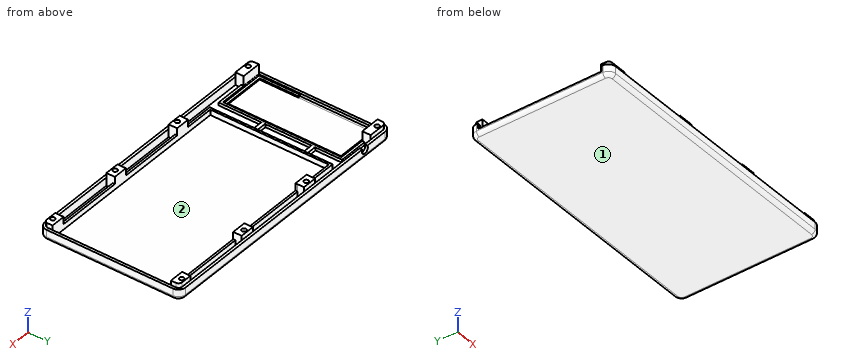
from build123d import *

# Parameters (mm, degrees)
ESQUISSE1_W             = 152.2
ESQUISSE1_H             = 78.4
BOSS_EXTRU_1_DEPTH      = 5.9
BOSS_EXTRU_2_DEPTH      = 1.4
BOSS_EXTRU_5_START      = 1.4
ESQUISSE1_5_R           = 1.25
BOSS_EXTRU_5_DEPTH      = 7
ESQUISSE1_5_W           = 8
ESQUISSE1_5_H           = 3.5
BOSS_EXTRU_5_2_DEPTH    = 7
BOSS_EXTRU_5_3_DEPTH    = 7
BOSS_EXTRU_5_4_DEPTH    = 7
BOSS_EXTRU_5_5_DEPTH    = 7
BOSS_EXTRU_5_6_DEPTH    = 7
BOSS_EXTRU_7_START      = 1.4
BOSS_EXTRU_7_DEPTH      = 3
CONG_1_R                = 4
CONG_4_R                = 2
BOSS_EXTRU_8_START      = 1.4
BOSS_EXTRU_8_DEPTH      = 0.75
BOSS_EXTRU_9_START      = 1.4
BOSS_EXTRU_9_DEPTH      = 1.65
BOSS_EXTRU_11_START     = 7
ESQUISSE4_R             = 1.25
BOSS_EXTRU_11_DEPTH     = 7
ESQUISSE5_W             = 6.6
ESQUISSE5_H             = 2
BOSS_EXTRU_12_DEPTH     = 2
CONG_3_R                = 2
ESQUISSE2_W             = 1.5
ESQUISSE2_H             = 68.8
ENL_V_MAT_EXTRU_1_DEPTH = 3
ENL_V_MAT_EXTRU_2_DEPTH = 1.5
ESQUISSE7_W             = 1.4
ESQUISSE7_H             = 41.680372202
ENL_V_MAT_EXTRU_3_DEPTH = 0.8
ESQUISSE8_W             = 7.99674486
ESQUISSE8_H             = 1.2
ESQUISSE8_W_2           = 8.000773141
ESQUISSE8_W_3           = 8
BOSS_EXTRU_13_DEPTH     = 4


with BuildPart() as part:
    # Esquisse1 → Boss.-Extru.1 (new body)
    with BuildSketch(Plane.XY):
        with Locations((74.6, 37.7)):
            Rectangle(ESQUISSE1_W, ESQUISSE1_H)
        with BuildLine():
            Line((0, 0), (147.2, 0))
            ThreePointArc((147.2, 0), (148.614213562, 0.585786438), (149.2, 2))
            Line((149.2, 2), (149.2, 73.4))
            ThreePointArc((149.2, 73.4), (148.614213562, 74.814213562), (147.2, 75.4))
            Line((147.2, 75.4), (0, 75.4))
            Line((0, 75.4), (0, 0))
        make_face(mode=Mode.SUBTRACT)
    extrude(amount=BOSS_EXTRU_1_DEPTH)

    # Esquisse1<4> → Boss.-Extru.2 (add)
    with BuildSketch(Plane.XY):
        with BuildLine():
            Line((0, 0), (147.2, 0))
            ThreePointArc((147.2, 0), (148.614213562, 0.585786438), (149.2, 2))
            Line((149.2, 2), (149.2, 73.4))
            ThreePointArc((149.2, 73.4), (148.614213562, 74.814213562), (147.2, 75.4))
            Line((147.2, 75.4), (0, 75.4))
            Line((0, 75.4), (0, 0))
        make_face()
    extrude(amount=BOSS_EXTRU_2_DEPTH)

    # Esquisse1<6> → Boss.-Extru.7 (add)
    with BuildSketch(Plane.XY.offset(BOSS_EXTRU_7_START)):
        Polygon((149.2, 70.7), (149.2, 71.9), (141.2, 71.9), (104.2, 71.9), (96.2, 71.9), (59.2, 71.9), (51.2, 71.9), (34, 71.9), (34, 37.7), (35.2, 37.7), (35.2, 70.7), align=None)
        Polygon((149.2, 3.5), (149.2, 4.7), (35.2, 4.7), (35.2, 37.7), (34, 37.7), (34, 3.5), (51.2, 3.5), (59.2, 3.5), (96.2, 3.5), (104.2, 3.5), (141.2, 3.5), align=None)
    extrude(amount=BOSS_EXTRU_7_DEPTH)

    # Congé1
    cong_1_edges = [part.edges().sort_by_distance(p)[0] for p in [
        (-1.5, 76.9, 2.95),
        (150.7, 76.9, 2.95),
        (150.7, -1.5, 2.95),
        (-1.5, -1.5, 2.95),
    ]]
    fillet(cong_1_edges, radius=CONG_1_R)

    # Congé4
    cong_4_edges = [part.edges().sort_by_distance(p)[0] for p in [
        (0, 75.4, 3.65),
        (0, 0, 3.65),
    ]]
    fillet(cong_4_edges, radius=CONG_4_R)

    # Esquisse1<7> → Boss.-Extru.8 (add)
    with BuildSketch(Plane.XY.offset(BOSS_EXTRU_8_START)):
        Polygon((24.6, 37.7), (26, 37.7), (26, 70.7), (0, 70.7), (0, 37.7), (1.4, 37.7), (1.4, 69.3), (24.6, 69.3), align=None)
        Polygon((26, 4.7), (26, 37.7), (24.6, 37.7), (24.6, 6.1), (1.4, 6.1), (1.4, 37.7), (0, 37.7), (0, 4.7), align=None)
    extrude(amount=BOSS_EXTRU_8_DEPTH)

    # Esquisse1<8> → Boss.-Extru.9 (add)
    with BuildSketch(Plane.XY.offset(BOSS_EXTRU_9_START)):
        Polygon((27.4, 3.3), (27.4, 72.1), (0, 72.1), (0, 70.7), (26, 70.7), (26, 4.7), (0, 4.7), (0, 3.3), align=None)
    extrude(amount=BOSS_EXTRU_9_DEPTH)

    # Esquisse4 → Boss.-Extru.11 (add)
    # profile 1 of 2: a face of its own
    with BuildSketch(Plane.XY.offset(1.4).offset(BOSS_EXTRU_11_START)):
        with BuildLine():
            Line((11, 75.4), (2, 75.4))
            ThreePointArc((2, 75.4), (0.585786438, 74.814213562), (0, 73.4))
            Line((0, 73.4), (0, 70.737356087))
            Line((0, 70.737356087), (11, 70.737356087))
            Line((11, 70.737356087), (11, 75.4))
        make_face()
        with Locations((4, 73.6)):
            Circle(ESQUISSE4_R, mode=Mode.SUBTRACT)
    # profile 2 of 2: a face of its own
    with BuildSketch(Plane.XY.offset(1.4).offset(BOSS_EXTRU_11_START)):
        with BuildLine():
            Line((0, 4.608067271), (11, 4.608067271))
            Line((11, 4.608067271), (11, 0))
            Line((11, 0), (2, 0))
            ThreePointArc((2, 0), (0.585786438, 0.585786438), (0, 2))
            Line((0, 2), (0, 4.608067271))
        make_face()
        with Locations((4, 1.8)):
            Circle(ESQUISSE4_R, mode=Mode.SUBTRACT)
    extrude(amount=-BOSS_EXTRU_11_DEPTH)

    # Esquisse5 → Boss.-Extru.12 (add)
    with BuildSketch(Plane.XY.offset(1.4)):
        with Locations((30.7, 56.329620473)):
            Rectangle(ESQUISSE5_W, ESQUISSE5_H)
        with Locations((30.7, 28.421993419)):
            Rectangle(ESQUISSE5_W, ESQUISSE5_H)
    extrude(amount=BOSS_EXTRU_12_DEPTH)

    # Congé3
    cong_3_edges = [part.edges().sort_by_distance(p)[0] for p in [
        (-1.5, 37.7, 0),
        (74.6, 76.9, 0),
        (150.7, 37.7, 0),
        (74.6, -1.5, 0),
        (149.528427125, 75.728427125, 0),
        (149.528427125, -0.328427125, 0),
        (-0.328427125, -0.328427125, 0),
        (-0.328427125, 75.728427125, 0),
    ]]
    fillet(cong_3_edges, radius=CONG_3_R)

    # Esquisse2 → Enlèv. mat.-Extru.1 (cut)
    with BuildSketch(Plane.XY.offset(5.9)):
        with Locations((-0.75, 37.7)):
            Rectangle(ESQUISSE2_W, ESQUISSE2_H)
    extrude(amount=-ENL_V_MAT_EXTRU_1_DEPTH, mode=Mode.SUBTRACT)

    # Esquisse6 → Enlèv. mat.-Extru.2 (cut)
    with BuildSketch(Plane(origin=(0, 76.9, 0), x_dir=(1, 0, 0), z_dir=(0, 1, 0))):
        with BuildLine():
            Line((17, -2.595457244), (17.25, -2.595457244))
            ThreePointArc((17.25, -2.595457244), (18.664213562, -3.181243681), (19.25, -4.595457244))
            Line((19.25, -4.595457244), (19.25, -4.845457244))
            ThreePointArc((19.25, -4.845457244), (18.664213562, -6.259670806), (17.25, -6.845457244))
            Line((17.25, -6.845457244), (17, -6.845457244))
            ThreePointArc((17, -6.845457244), (15.585786438, -6.259670806), (15, -4.845457244))
            Line((15, -4.845457244), (15, -4.595457244))
            ThreePointArc((15, -4.595457244), (15.585786438, -3.181243681), (17, -2.595457244))
        make_face()
    extrude(amount=-ENL_V_MAT_EXTRU_2_DEPTH, mode=Mode.SUBTRACT)

    # Esquisse7 → Enlèv. mat.-Extru.3 (cut)
    with BuildSketch(Plane.XY.offset(2.15)):
        with Locations((0.7, 48.459813899)):
            Rectangle(ESQUISSE7_W, ESQUISSE7_H)
    extrude(amount=-ENL_V_MAT_EXTRU_3_DEPTH, mode=Mode.SUBTRACT)



with BuildPart() as body_2:
    # Esquisse1<5> → Boss.-Extru.5 (new body)
    with BuildSketch(Plane.XY.offset(BOSS_EXTRU_5_START)):
        with BuildLine():
            Line((141.2, 71.9), (149.2, 71.9))
            Line((149.2, 71.9), (149.2, 73.4))
            ThreePointArc((149.2, 73.4), (148.614213562, 74.814213562), (147.2, 75.4))
            Line((147.2, 75.4), (141.2, 75.4))
            Line((141.2, 75.4), (141.2, 71.9))
        make_face()
        with Locations(Location((145.2, 73.6, 0), (0, 0, 180))):
            Circle(ESQUISSE1_5_R, mode=Mode.SUBTRACT)
    extrude(amount=BOSS_EXTRU_5_DEPTH)


with BuildPart() as body_3:
    # Esquisse1<5> → Boss.-Extru.5 2 (new body)
    with BuildSketch(Plane.XY.offset(BOSS_EXTRU_5_START)):
        with Locations((100.2, 73.65)):
            Rectangle(ESQUISSE1_5_W, ESQUISSE1_5_H)
        with Locations(Location((100.2, 73.6, 0), (0, 0, 180))):
            Circle(ESQUISSE1_5_R, mode=Mode.SUBTRACT)
    extrude(amount=BOSS_EXTRU_5_2_DEPTH)


with BuildPart() as body_4:
    # Esquisse1<5> → Boss.-Extru.5 3 (new body)
    with BuildSketch(Plane.XY.offset(BOSS_EXTRU_5_START)):
        with BuildLine():
            Line((149.2, 2), (149.2, 3.5))
            Line((149.2, 3.5), (141.2, 3.5))
            Line((141.2, 3.5), (141.2, 0))
            Line((141.2, 0), (147.2, 0))
            ThreePointArc((147.2, 0), (148.614213562, 0.585786438), (149.2, 2))
        make_face()
        with Locations(Location((145.2, 1.8, 0), (0, 0, 180))):
            Circle(ESQUISSE1_5_R, mode=Mode.SUBTRACT)
    extrude(amount=BOSS_EXTRU_5_3_DEPTH)


with BuildPart() as body_5:
    # Esquisse1<5> → Boss.-Extru.5 4 (new body)
    with BuildSketch(Plane.XY.offset(BOSS_EXTRU_5_START)):
        with Locations((55.2, 73.65)):
            Rectangle(ESQUISSE1_5_W, ESQUISSE1_5_H)
        with Locations(Location((55.2, 73.6, 0), (0, 0, 180))):
            Circle(ESQUISSE1_5_R, mode=Mode.SUBTRACT)
    extrude(amount=BOSS_EXTRU_5_4_DEPTH)


with BuildPart() as body_6:
    # Esquisse1<5> → Boss.-Extru.5 5 (new body)
    with BuildSketch(Plane.XY.offset(BOSS_EXTRU_5_START)):
        with Locations((100.2, 1.75)):
            Rectangle(ESQUISSE1_5_W, ESQUISSE1_5_H)
        with Locations(Location((100.2, 1.8, 0), (0, 0, 180))):
            Circle(ESQUISSE1_5_R, mode=Mode.SUBTRACT)
    extrude(amount=BOSS_EXTRU_5_5_DEPTH)


with BuildPart() as body_7:
    # Esquisse1<5> → Boss.-Extru.5 6 (new body)
    with BuildSketch(Plane.XY.offset(BOSS_EXTRU_5_START)):
        with Locations((55.2, 1.75)):
            Rectangle(ESQUISSE1_5_W, ESQUISSE1_5_H)
        with Locations(Location((55.2, 1.8, 0), (0, 0, 180))):
            Circle(ESQUISSE1_5_R, mode=Mode.SUBTRACT)
    extrude(amount=BOSS_EXTRU_5_6_DEPTH)


with BuildPart() as part_1:
    add(part.part)

    add(body_2.part)  # Boss.-Extru.13 merges body 2

    add(body_3.part)  # Boss.-Extru.13 merges body 3

    add(body_4.part)  # Boss.-Extru.13 merges body 4

    add(body_5.part)  # Boss.-Extru.13 merges body 5

    add(body_6.part)  # Boss.-Extru.13 merges body 6

    add(body_7.part)  # Boss.-Extru.13 merges body 7
    # Esquisse8 → Boss.-Extru.13 (add)
    with BuildSketch(Plane.XY.offset(4.4)):
        with Locations((55.19837243, 71.3)):
            Rectangle(ESQUISSE8_W, ESQUISSE8_H)
        with Locations((100.19961343, 71.3)):
            Rectangle(ESQUISSE8_W_2, ESQUISSE8_H)
        with Locations((145.2, 71.3)):
            Rectangle(ESQUISSE8_W_3, ESQUISSE8_H)
        with Locations((145.2, 4.1)):
            Rectangle(ESQUISSE8_W_3, ESQUISSE8_H)
        with Locations((100.19961343, 4.1)):
            Rectangle(ESQUISSE8_W_2, ESQUISSE8_H)
        with Locations((55.2, 4.1)):
            Rectangle(ESQUISSE8_W_3, ESQUISSE8_H)
    extrude(amount=BOSS_EXTRU_13_DEPTH)


solid = part_1.part
Geometry: final body of the model. Coordinates: model frame, mm. Face numbers are marked on the shaded views. Coordinates: 2 decimals unless noted, no trailing zeros. Write each loop counter-clockwise with the first axis right and the second up, starting at its lowest first coordinate (ties: lowest second). Pieces come first, ordered by that corner, then holes. Notation, with made-up numbers: (29.5, -15) - (67.5, -15) arc R24 cw to (67.5, 18) - close; hole circle Ø10 at (-24.75, 49.5). An arc over 180 degrees is marked (long way). Return JSON: item names as keys, results as strings.
Item 1: Pin query (flat end, axial travel): pin 1 Ø12 at (x, y) = (43.5, 40.5) entering from +Z; pin 2 Ø3 at (x, y) = (145.2, 73.6) entering from +Z; pin 3 Ø1 at (y, z) = (71.5, 7) entering from +X; pin 4 Ø0.6 at (x, y) = (31, 28.5) entering from +Z. Return the tip coordinate at first contact, or that it passes through.
Completed:
{"pin 1": "stops at z = 1.4", "pin 2": "stops at z = 8.4", "pin 3": "stops at x = 149.2", "pin 4": "stops at z = 3.4"}
Item 2: Line query: L1, parallel to Y at x = 100.2, z = 7; L2, parallel to Y at x = 75.5, z = 3.25; L3, parallel to X at y = 24, z = 2.5. Output: solid intervals per line, ascending.
Completed:
{"L1": "y = 0 to 0.55, 3.05 to 4.7, 70.7 to 72.35, 74.85 to 75.4", "L2": "y = -1.5 to 0, 3.5 to 4.7, 70.7 to 71.9, 75.4 to 76.9", "L3": "x = -1.5 to 0, 26 to 27.4, 34 to 35.2, 149.2 to 150.7"}
Item 3: Section query C-C (y = 18.5). Output: boundary loops of the cut face in (x, z).
Completed:
{"outline": "(-1.5, 2) arc R2 ccw to (0.5, 0) - (148.7, 0) arc R2 ccw to (150.7, 2) - (150.7, 5.9) - (149.2, 5.9) - (149.2, 1.4) - (35.2, 1.4) - (35.2, 4.4) - (34, 4.4) - (34, 1.4) - (27.4, 1.4) - (27.4, 3.05) - (26, 3.05) - (26, 2.15) - (24.6, 2.15) - (24.6, 1.4) - (1.4, 1.4) - (1.4, 2.15) - (0, 2.15) - (0, 2.9) - (-1.5, 2.9) - close"}
Item 4: Pull-direction query (Y, two-part tool) for the marked faces 1 and 2; classes: +Y half, -Y half, draft (parallel to the pull), parting line (faces both ways), or undercut.
Completed:
{"face 1": "draft", "face 2": "undercut"}
Item 5: Section query B-B (x = 124.5). Output: boundary loops of the cut face in (y, z).
Completed:
{"outline": "(-1.5, 2) arc R2 ccw to (0.5, 0) - (74.9, 0) arc R2 ccw to (76.9, 2) - (76.9, 5.9) - (75.4, 5.9) - (75.4, 1.4) - (71.9, 1.4) - (71.9, 4.4) - (70.7, 4.4) - (70.7, 1.4) - (4.7, 1.4) - (4.7, 4.4) - (3.5, 4.4) - (3.5, 1.4) - (0, 1.4) - (0, 5.9) - (-1.5, 5.9) - close"}
Item 6: Section query A-A (y = 36). Output: boundary loops of the cut face in (x, z).
Completed:
{"outline": "(-1.5, 2) arc R2 ccw to (0.5, 0) - (148.7, 0) arc R2 ccw to (150.7, 2) - (150.7, 5.9) - (149.2, 5.9) - (149.2, 1.4) - (35.2, 1.4) - (35.2, 4.4) - (34, 4.4) - (34, 1.4) - (27.4, 1.4) - (27.4, 3.05) - (26, 3.05) - (26, 2.15) - (24.6, 2.15) - (24.6, 1.4) - (1.4, 1.4) - (1.4, 1.35) - (0, 1.35) - (0, 2.9) - (-1.5, 2.9) - close"}
